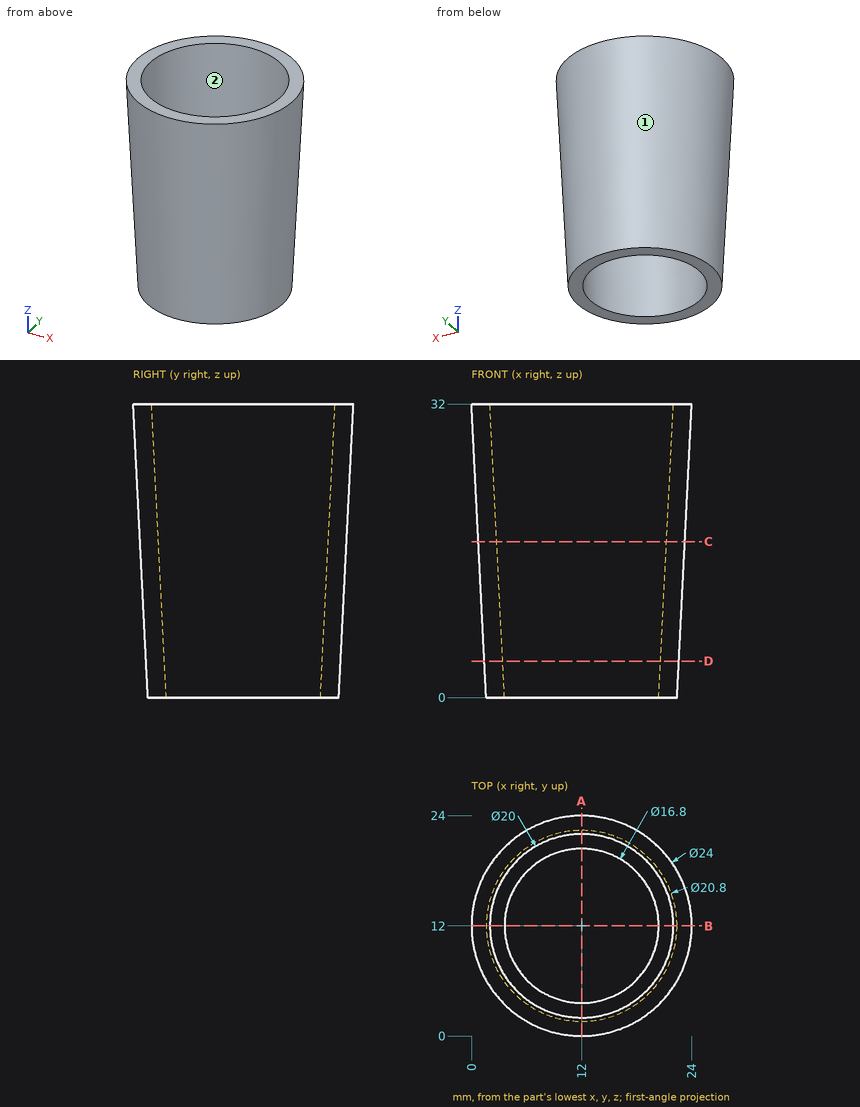
Input: dimensioned drawing with shaded views. Units: mm. Origin: part minimum x, y, z. Give positions to 0.01 mm unless a question says otherwise; leave off trailing zeros. Write each loop counter-clockwise with the first axis right and the second up, starting at its lowest first coordinate (ties: lowest second). Pieces come first, ordered by that corner, then holes. Notation, with made-up numbers: M 22.5,38 L 58.5,38 A33 ccw 58.5,68 Z; hole C -2.5,50.5 d2. An arc over 180 degrees is marked long. Return JSON: item names as keys, results as strings. Group by question number.
1) Cut plane C-C, the plane z = 17. Output: boundary loops of the cut face in (x, y), plus the area to 3 significant figures.
2) Material intervals for line 1 along X through (y, z) = (7, 21.5); line 2 along X through (y, z) = (19.5, 17); line 3 along Y through (x, z) = (14.5, 28.5), sorted ascending. Write a range as [from, to].
3) Cut plane D-D, the plane z = 4. Output: boundary loops of the cut face in (x, y).
4) Pull-direction query (Y, two-part tool) for the marked faces 1 and 2; classes: pulls with the +Y half, pulls with the -Y half, needs draft (parallel to the pull), parting line crosses it, or undercut.
5) Cut plane A-A, the plane x = 12. Output: boundary loops of the cut face in (y, z).
6) Pin query (flat end, axial travel): P1, Ø6, axis at x = 11.5, z = 24, coming from the +Y side; P2, Ø4, axis at y = 10.5, z = 19.5, coming from the +X side; P3, Ø8, axis at x = 6, z = 8, coming from the +Y side. Return the tip coordinate at first contact, or that it passes through.
Recorded:
{
 "1": {"outline": "C 12,12 d22.5; hole C 12,12 d18.5", "area": "129 mm²"},
 "2": {"line 1": "x = [1.67, 3.95], [20.05, 22.33]", "line 2": "x = [3.61, 6.59], [17.41, 20.39]", "line 3": "y = [0.44, 2.5], [21.5, 23.56]"},
 "3": {"outline": "C 12,12 d21.2; hole C 12,12 d17.2"},
 "4": {"face 1": "parting line crosses it", "face 2": "undercut"},
 "5": {"outline": "M 0,32 L 1.6,0 L 3.6,0 L 2,32 Z; M 20.4,0 L 22.4,0 L 24,32 L 22,32 Z"},
 "6": {"P1": "stops at y = 23.75", "P2": "stops at x = 23.45", "P3": "stops at y = 22.64"}
}
